Geometry: final body of the model. Coordinates: model frame, mm. Face numbers are marked on the shaded views. A direction names the side the tool comes from. Coordinates: 2 decimals unless noted, no trailing zeros. Loops run counter-clockwise (first coordinate to the right, second up) from the corner with the lowest first, then second, coordinate; pieces in that order, holes last. Notation, with made-up numbers: (-26, 79) - (27, 79) arc R27 ccw to (27, 99) - close; hole circle Ø7 at (38, 22.5). An arc over 180 degrees is marked (long way). Answer in a Markdown table with one row per item.
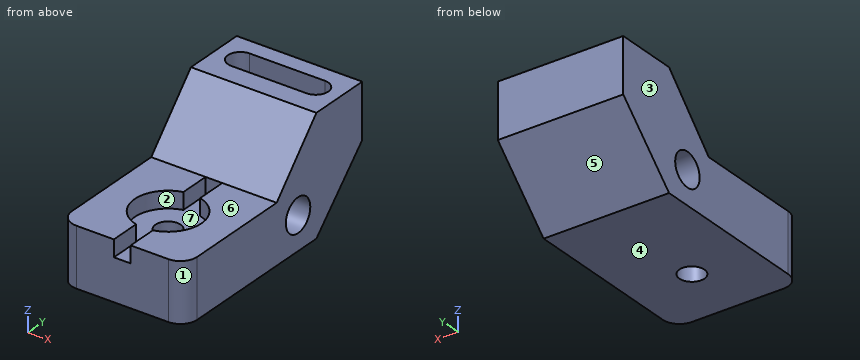
from build123d import *

# Parameters (mm, degrees)
F0_R           = 10.16
F1_DEPTH       = 38.1
F3_DEPTH       = 27.94
F6_D           = 15.24
F6_CBORE_D     = 40.64
F6_CBORE_DEPTH = 10.16
F4_W           = 10.16
F4_H           = 10.16
F7_DEPTH       = 76.2
F8_R           = 10.16


with BuildPart() as f1:
    # F0 (on Right) → F1 (new body, symmetric)
    with BuildSketch(Plane.YZ):
        Polygon((-109.22, 0), (0, 0), (38.1, 38.1), (38.1, 71.12), (0, 71.12), (-33.02, 35.56), (-109.22, 35.56), align=None)
        with Locations((-15.24, 20.32)):
            Circle(F0_R, mode=Mode.SUBTRACT)
    extrude(amount=F1_DEPTH, both=True)

    # F2 (on face) → F3 (cut)
    with BuildSketch(Plane.XY.offset(71.12)):
        with BuildLine():
            Line((22.86, 27.94), (-22.86, 27.94))
            ThreePointArc((-22.86, 27.94), (-30.48, 20.32), (-22.86, 12.7))
            Line((-22.86, 12.7), (22.86, 12.7))
            ThreePointArc((22.86, 12.7), (30.48, 20.32), (22.86, 27.94))
        make_face()
    extrude(amount=-F3_DEPTH, mode=Mode.SUBTRACT)

    # F6 (through all)
    with Locations(Plane.XY.offset(35.56)):
        with Locations((0, -71.12)):
            CounterBoreHole(F6_D / 2, F6_CBORE_D / 2, F6_CBORE_DEPTH)

    # F4 (on face) → F7 (cut)
    with BuildSketch(Plane.XZ.offset(109.22)):
        with Locations((0, 30.48)):
            Rectangle(F4_W, F4_H)
    extrude(amount=-F7_DEPTH, mode=Mode.SUBTRACT)

    # F8
    f8_edges = [f1.edges().sort_by_distance(p)[0] for p in [
        (-38.1, -109.22, 17.78),
        (38.1, -109.22, 17.78),
    ]]
    fillet(f8_edges, radius=F8_R)


solid = f1.part
(1) Cut plane C-C on y = -71.12. Output: boundary loops of the cut face in (x, z), then the cut area to 3 significant figures.
Verdict:
| item | result |
|---|---|
| outline | (-38.1, 0) - (-7.62, 0) - (-7.62, 25.4) - (-20.32, 25.4) - (-20.32, 35.56) - (-38.1, 35.56) - close; (7.62, 0) - (38.1, 0) - (38.1, 35.56) - (20.32, 35.56) - (20.32, 25.4) - (7.62, 25.4) - close |
| area | 1,910 mm² |
(2) Ray query, probe 1 along Y at (x, z) = (5, 22); probe 2 along Y at (x, z) = (0, 19); probe 3 along Y at (x, z) = (0, 54). Return the intervals inside material, ascending.
Verdict:
| item | result |
|---|---|
| probe 1 | y = -109.22 to -76.87, -65.37 to -25.26, -5.22 to 22 |
| probe 2 | y = -109.22 to -78.74, -63.5 to -25.31, -5.17 to 19 |
| probe 3 | y = -15.9 to 12.7, 27.94 to 38.1 |
(3) Cut plane A-A on x = 0. Output: boundary loops of the cut face in (y, z).
Verdict:
| item | result |
|---|---|
| outline | (-109.22, 0) - (-78.74, 0) - (-78.74, 25.4) - (-109.22, 25.4) - close; (-63.5, 0) - (0, 0) - (38.1, 38.1) - (38.1, 71.12) - (27.94, 71.12) - (27.94, 43.18) - (12.7, 43.18) - (12.7, 71.12) - (0, 71.12) - (-33.02, 35.56) - (-33.02, 25.4) - (-63.5, 25.4) - close; hole circle Ø20.32 at (-15.24, 20.32) |
(4) Cut plane D-D on z = 32.5. Output: boundary loops of the cut face in (x, y).
Verdict:
| item | result |
|---|---|
| outline | (-38.1, -99.06) arc R10.16 ccw to (-27.94, -109.22) - (-5.08, -109.22) - (-5.08, -90.79) arc R20.32 cw to (-5.08, -51.45) - (-5.08, -33.02) - (5.08, -33.02) - (5.08, -51.45) arc R20.32 cw to (5.08, -90.79) - (5.08, -109.22) - (27.94, -109.22) arc R10.16 ccw to (38.1, -99.06) - (38.1, 32.5) - (-38.1, 32.5) - close |
(5) Cut plane B-B on z = 20.32. Output: boundary loops of the cut face in (x, y).
Verdict:
| item | result |
|---|---|
| outline | (-38.1, -99.06) arc R10.16 ccw to (-27.94, -109.22) - (27.94, -109.22) arc R10.16 ccw to (38.1, -99.06) - (38.1, -25.4) - (-38.1, -25.4) - close; (-38.1, -5.08) - (38.1, -5.08) - (38.1, 20.32) - (-38.1, 20.32) - close; hole circle Ø15.24 at (0, -71.12) |
(6) Pull-direction query (X, two-part tool) for the marked faces 1, 2, 3 and 4; classes: pulls with the +X half, pulls with the -X half, needs draft (parallel to the pull), parting line crosses it, or undercut.
Verdict:
| item | result |
|---|---|
| face 1 | pulls with the +X half |
| face 2 | undercut |
| face 3 | pulls with the -X half |
| face 4 | needs draft |
(7) First-contact query: pin 1 Ø12 at (x, y) = (0, -71.12) entering from +Z; pin 2 Ø20.5 at (x, y) = (-7, -73) entering from +Z; pin 3 Ø16.5 at (x, y) = (21, -73.5) entering from +Z; pin 4 Ø22.5 at (x, z) = (6.5, 56) entering from -Y. Flat tips, straight axial feed; report the tip coordinate or a pass-through.
Verdict:
| item | result |
|---|---|
| pin 1 | passes through |
| pin 2 | stops at z = 25.4 |
| pin 3 | stops at z = 35.56 |
| pin 4 | stops at y = -24.49 |
(8) Access query for the marked faces 5, 6 and 7. Directions: +Z, -Z, +X, -X, +Y, -Y. A direction counts if a zero-diameter tool reaches every point of the face in a straight line with its end or side. Return the directions, or none.
Verdict:
| item | result |
|---|---|
| face 5 | -Z, +X, -X, +Y |
| face 6 | +Z, +X, -X, -Y |
| face 7 | +Z |
